```python
from build123d import *

# Parameters (mm, degrees)
SKETCH1_W                       = 12.7
SKETCH1_H                       = 50.8
EXTRUDE1_DEPTH                  = 3.175
F_1_4_0_25_DIAMETER_HOLE1_D     = 6.35
F_1_4_0_25_DIAMETER_HOLE1_DEPTH = 6.35
F_1_4_0_25_DIAMETER_HOLE1_TIP   = 1.907732465
FILLET1_R                       = 5.08


with BuildPart() as part:
    # Sketch1 → Extrude1 (new body)
    with BuildSketch(Plane.XY):
        Rectangle(SKETCH1_W, SKETCH1_H)
    extrude(amount=EXTRUDE1_DEPTH)

    # 1/4 (0.25) Diameter Hole1
    with Locations(Plane(origin=(0, 19.05, 3.175), x_dir=(1, 0, 0), z_dir=(0, 0, 1))):
        with Locations((0, 0)):
            Hole(F_1_4_0_25_DIAMETER_HOLE1_D / 2, depth=F_1_4_0_25_DIAMETER_HOLE1_DEPTH)
            with Locations((0, 0, -(F_1_4_0_25_DIAMETER_HOLE1_DEPTH + F_1_4_0_25_DIAMETER_HOLE1_TIP / 2))):  # 118° drill point
                Cone(0, F_1_4_0_25_DIAMETER_HOLE1_D / 2, F_1_4_0_25_DIAMETER_HOLE1_TIP, mode=Mode.SUBTRACT)

    # Fillet1
    fillet1_edges = [part.edges().sort_by_distance(p)[0] for p in [
        (-6.35, 25.4, 1.5875),
        (6.35, 25.4, 1.5875),
    ]]
    fillet(fillet1_edges, radius=FILLET1_R)


solid = part.part
```
For this review, take the finished solid that the model builds, in its own axes (mm). Give positions to 0.01 mm unless a question says otherwise; leave off trailing zeros. Write each loop counter-clockwise with the first axis right and the second up, starting at its lowest first coordinate (ties: lowest second). Pieces come first, ordered by that corner, then holes.
Item 1: Take a section at B-B (x = 0). Give the boundary of the cut face in (y, z) (3 decimals).
Item 2: Take a section at A-A (z = 2.2). Give the boundary of the cut face in (x, y) (3 decimals).
Item 3: Take a section at C-C (y = 19.05). Give the boundary of the cut face in (x, z) (3 decimals).
Item 4: Wall thickness on probe 1 along Y at (x, z) = (0, 0.95) (3 decimals); probe 2 along X at (y, z) = (18, 1.55); probe 3 along Y at (x, z) = (-1, 0.9): over which ranges is each line inside the solid? List them lowest first.
Item 5: Insertion check: P1, Ø5.5, axis at x = 0, y = 19.05, coming from the +Z side. The pin has a flat end and moves straight along its axis. Give the tip position at first contact, or say it passes through.
Item 6: Take a section at D-D (x = 4.75). Give the boundary of the cut face in (y, z) (3 decimals), and give its area (3 significant figures).
Established:
1. outline: (-25.4, 0) - (15.875, 0) - (15.875, 3.175) - (-25.4, 3.175) - close; (22.225, 0) - (25.4, 0) - (25.4, 3.175) - (22.225, 3.175) - close
2. outline: (-6.35, -25.4) - (6.35, -25.4) - (6.35, 20.32) arc R5.08 ccw to (1.27, 25.4) - (-1.27, 25.4) arc R5.08 ccw to (-6.35, 20.32) - close; hole circle Ø6.35 at (0, 19.05)
3. outline: (-6.35, 0) - (-3.175, 0) - (-3.175, 3.175) - (-6.35, 3.175) - close; (3.175, 0) - (6.35, 0) - (6.35, 3.175) - (3.175, 3.175) - close
4. probe 1: y = -25.4 to 15.875, 22.225 to 25.4
4. probe 2: x = -6.35 to -3, 3 to 6.35
4. probe 3: y = -25.4 to 16.04, 22.06 to 25.4
5. P1: passes through
6. outline: (-25.4, 0) - (24.021, 0) - (24.021, 3.175) - (-25.4, 3.175) - close
6. area: 157 mm2
